For this review, take the finished solid that the model builds, in its own axes (mm). A direction names the side the tool comes from. Round coordinates to 2 decimals unless told otherwise and drop trailing zeros. Loops run counter-clockwise (first coordinate to the right, second up) from the corner with the lowest first, then second, coordinate; pieces in that order, holes last. Notation, with made-up numbers: (-8.5, 61) -> (40.5, 61) arc R27 ccw to (40.5, 94) -> close; hole circle Ø8 at (55, 70.5). An arc over 180 degrees is marked (long way). One line per question, with ' | ' between items. Start each with the question number.
1. Draft analysis for pull direction Y (two halves, no side actions). For faces 3 (the face through (0, 4.762, 1)), 4 (the face through (3.446, -2.356, 1.565)), 5 (the face through (0, 0, 0)), state which applies: pulls with the +Y half, pulls with the -Y half, needs draft (parallel to the pull), parting line crosses it, or undercut.
2. Consider section D-D (x = 0.5). Write out the cut boundary in (y, z).
3. For faces 1 (the face through (0, -4.762, 1)), 2 (the face through (5.34, -2.64, 2.77)), list the 3-axis set-ups (+Z, -Z, +X, -X, +Y, -Y) from which the entire face can be reached by the end or side of a thin tool; tool diameter is ignored.
4. Wall thickness on line 1 along Z through (x, y) = (-6.75, 2.25); line 2 along X through (y, z) = (-1, 3); line 3 along Y through (x, z) = (2.5, 2.65): over which ranges is each line inside the solid? List them lowest first.
5. Consider section B-B (x = 5). Write out the cut boundary in (y, z) (1 decimal), and give its area (3 significant figures).
6. For pin 1 Ø1.5 at (y, z) = (-1.5, 2) entering from -X, flat-tipped, find the tip position at first contact; note if it passes through.
7. Consider section A-A (y = 0). Write out the cut boundary in (x, z) (1 decimal).
```python
from build123d import *

# Parameters (mm, degrees)
SKETCH1_R      = 2.413
EXTRUDE1_DEPTH = 2.38125
SKETCH2_R      = 2.9765625
SKETCH2_R_2    = 2.413
EXTRUDE2_DEPTH = 0.79375


with BuildPart() as part:
    # Sketch1 → Extrude1 (new body)
    with BuildSketch(Plane.XY):
        with BuildLine():
            Line((-6.35, 4.7625), (6.35, 4.7625))
            ThreePointArc((6.35, 4.7625), (7.9375, 0), (6.35, -4.7625))
            Line((6.35, -4.7625), (-6.35, -4.7625))
            ThreePointArc((-6.35, -4.7625), (-7.9375, 0), (-6.35, 4.7625))
        make_face()
        with Locations((3.96875, 0)):
            Circle(SKETCH1_R, mode=Mode.SUBTRACT)
    extrude(amount=EXTRUDE1_DEPTH)

    # Sketch2 → Extrude2 (add)
    with BuildSketch(Plane.XY.offset(2.38125)):
        with Locations((3.96875, 0)):
            Circle(SKETCH2_R)
        with Locations((3.96875, 0)):
            Circle(SKETCH2_R_2, mode=Mode.SUBTRACT)
    extrude(amount=EXTRUDE2_DEPTH)


solid = part.part
```
Answer block:
1) face 3: pulls with the +Y half | face 4: undercut | face 5: needs draft
2) outline: (-4.76, 0) -> (4.76, 0) -> (4.76, 2.38) -> (-4.76, 2.38) -> close
3) face 1: +Z, -Z, +X, -X, -Y | face 2: +Z
4) line 1: z = 0 to 2.38 | line 2: x = 1.17 to 1.77, 6.16 to 6.77 | line 3: y = -2.59 to -1.91, 1.91 to 2.59
5) outline: (-4.8, 0) -> (-2.2, 0) -> (-2.2, 3.2) -> (-2.8, 3.2) -> (-2.8, 2.4) -> (-4.8, 2.4) -> close; (2.2, 0) -> (4.8, 0) -> (4.8, 2.4) -> (2.8, 2.4) -> (2.8, 3.2) -> (2.2, 3.2) -> close | area: 13.3 mm2
6) pin 1: stops at x = -7.9
7) outline: (-7.9, 0) -> (1.6, 0) -> (1.6, 3.2) -> (1, 3.2) -> (1, 2.4) -> (-7.9, 2.4) -> close; (6.4, 0) -> (7.9, 0) -> (7.9, 2.4) -> (6.9, 2.4) -> (6.9, 3.2) -> (6.4, 3.2) -> close
